```python
from build123d import *

# Parameters (mm, degrees)
SKETCH1_W                 = 146.05
SKETCH1_H                 = 101.6
BOSS_EXTRUDE1_DEPTH       = 1.5875
FILLET1_R                 = 6.35
F_4_CLEARANCE_HOLE1_D     = 3.2639
F_4_CLEARANCE_HOLE1_DEPTH = 50.8
F_4_CLEARANCE_HOLE1_TIP   = 0.980574487
M3_CLEARANCE_HOLE1_D      = 3.4
F_4_CLEARANCE_HOLE2_D     = 3.2639
F_2_CLEARANCE_HOLE1_D     = 2.4384


with BuildPart() as part:
    # Sketch1 → Boss-Extrude1 (new body)
    with BuildSketch(Plane(origin=(0, 0, 0), x_dir=(1, 0, 0), z_dir=(0, 1, 0))):
        Rectangle(SKETCH1_W, SKETCH1_H)
    extrude(amount=BOSS_EXTRUDE1_DEPTH)

    # Fillet1
    fillet1_edges = [part.edges().sort_by_distance(p)[0] for p in [
        (73.025, 0.79375, 50.8),
        (-73.025, 0.79375, 50.8),
        (-73.025, 0.79375, -50.8),
        (73.025, 0.79375, -50.8),
    ]]
    fillet(fillet1_edges, radius=FILLET1_R)

    # #4 Clearance Hole1
    with Locations(Plane(origin=(0, 1.5875, 0), x_dir=(-1, 0, 0), z_dir=(0, 1, 0))):
        with Locations((-66.675, 44.45), (-66.675, -44.45), (66.675, -44.45), (66.675, 44.45)):
            Hole(F_4_CLEARANCE_HOLE1_D / 2, depth=F_4_CLEARANCE_HOLE1_DEPTH)
            with Locations((0, 0, -(F_4_CLEARANCE_HOLE1_DEPTH + F_4_CLEARANCE_HOLE1_TIP / 2))):  # 118° drill point
                Cone(0, F_4_CLEARANCE_HOLE1_D / 2, F_4_CLEARANCE_HOLE1_TIP, mode=Mode.SUBTRACT)

    # M3 Clearance Hole1 (through all)
    with Locations(Plane(origin=(0, 1.5875, 0), x_dir=(-1, 0, 0), z_dir=(0, 1, 0))):
        with Locations((7.62, -38.1), (-53.975, -38.1), (7.62, 38.1), (-53.975, 38.1)):
            Hole(M3_CLEARANCE_HOLE1_D / 2)

    # #4 Clearance Hole2 (through all)
    with Locations(Plane(origin=(0, 1.5875, 0), x_dir=(-1, 0, 0), z_dir=(0, 1, 0))):
        with Locations((-69.215, 0), (-69.215, 34.925), (-69.215, -34.925)):
            Hole(F_4_CLEARANCE_HOLE2_D / 2)

    # #2 Clearance Hole1 (through all)
    with Locations(Plane.XZ):
        with Locations((-66.3194, -25.4), (-22.5806, -25.4), (-65.0875, 38.3794), (-23.8125, 38.3794)):
            Hole(F_2_CLEARANCE_HOLE1_D / 2)


solid = part.part
```
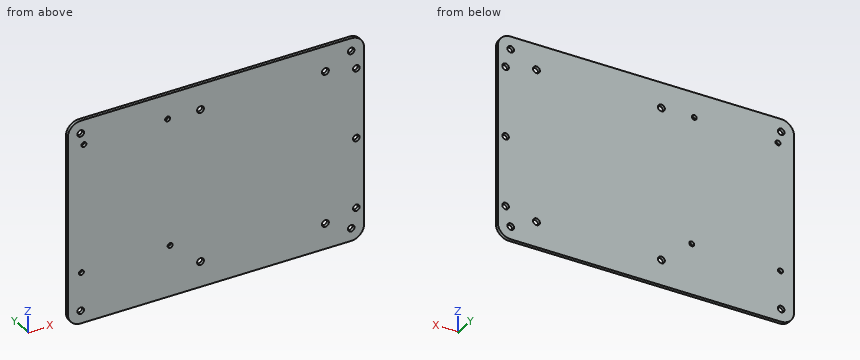
Verification items for the finished model (mm, model axes). Round coordinates to 2 decimals unless told otherwise and drop trailing zeros. Write each loop counter-clockwise with the first axis right and the second up, starting at its lowest first coordinate (ties: lowest second). Pieces come first, ordered by that corner, then holes. Notation, with made-up numbers: (47.25, 26) - (55.25, 26) arc R24 cw to (55.25, 55) - close; hole circle Ø4 at (86, 18). An arc over 180 degrees is marked (long way). Answer as a JSON object with one key per item and string values. Group by question number.
Q1. Go/stop test with a flat-tipped pin: pin 1 Ø2 at (x, z) = (-23.81, 38.38) entering from -Y. Record where the tip stops, or that it passes through.
Q2. Section check A-A, the plane z = 0. Enter the section's corners in (x, y) (1 decimal).
Q3. Thickness scan on line 1 (Z direction, x = -7.62, y = 0.9); line 2 (X direction, y = 1.4, z = -37) (3 decimals); line 3 (X direction, y = 0.6, z = -38) (3 decimals). Record the ranges inside material, lowest first.
Q4. Section check B-B, the plane x = -7.62. Enter the section's corners in (y, z).
Found:
{
 "1": {"pin 1": "passes through"},
 "2": {"outline": "(-73, 0) - (67.6, 0) - (67.6, 1.6) - (-73, 1.6) - close; (70.8, 0) - (73, 0) - (73, 1.6) - (70.8, 1.6) - close"},
 "3": {"line 1": "z = -50.8 to -39.8, -36.4 to 36.4, 39.8 to 50.8", "line 2": "x = -73.025 to -8.916, -6.324 to 52.679, 55.271 to 73.025", "line 3": "x = -73.025 to -9.317, -5.923 to 52.278, 55.672 to 73.025"},
 "4": {"outline": "(0, -50.8) - (1.59, -50.8) - (1.59, -39.8) - (0, -39.8) - close; (0, -36.4) - (1.59, -36.4) - (1.59, 36.4) - (0, 36.4) - close; (0, 39.8) - (1.59, 39.8) - (1.59, 50.8) - (0, 50.8) - close"}
}
